```python
from build123d import *

# Parameters (mm, degrees)
SKETCH1_W           = 150
SKETCH1_H           = 40
BOSS_EXTRUDE1_DEPTH = 2
SKETCH2_W           = 150
SKETCH2_H           = 2
BOSS_EXTRUDE2_DEPTH = 40
BOSS_EXTRUDE3_DEPTH = 390
CUT_EXTRUDE1_DEPTH  = 10
CUT_EXTRUDE2_DEPTH  = 10


with BuildPart() as part:
    # Sketch1 → Boss-Extrude1 (new body)
    with BuildSketch(Plane(origin=(0, 0, 0), x_dir=(1, 0, 0), z_dir=(0, 1, 0))):
        Rectangle(SKETCH1_W, SKETCH1_H)
    extrude(amount=BOSS_EXTRUDE1_DEPTH)

    # Sketch2 → Boss-Extrude2 (add)
    with BuildSketch(Plane(origin=(0, 2, 0), x_dir=(1, 0, 0), z_dir=(0, 1, 0))):
        with Locations((0, -19)):
            Rectangle(SKETCH2_W, SKETCH2_H)
    extrude(amount=BOSS_EXTRUDE2_DEPTH)

    # Sketch5 → Boss-Extrude3 (add)
    with BuildSketch(Plane(origin=(75, 0, 0), x_dir=(0, 0, -1), z_dir=(1, 0, 0))):
        Polygon((-20, 0), (20, 0), (20, 2), (-18, 2), (-18, 42), (-20, 42), align=None)
    extrude(amount=BOSS_EXTRUDE3_DEPTH)

    # Sketch6 → Cut-Extrude1 (cut)
    with BuildSketch(Plane.XZ):
        with BuildLine():
            Line((7.420621343, 6.493750786), (43.697093864, 6.493750786))
            ThreePointArc((43.697093864, 6.493750786), (50.190844651, 0), (43.697093864, -6.493750786))
            Line((43.697093864, -6.493750786), (7.420621343, -6.493750786))
            ThreePointArc((7.420621343, -6.493750786), (0.926870557, 0), (7.420621343, 6.493750786))
        make_face()
        with BuildLine():
            Line((-57.579378657, 6.493750786), (-21.302906136, 6.493750786))
            ThreePointArc((-21.302906136, 6.493750786), (-14.809155349, 0), (-21.302906136, -6.493750786))
            Line((-21.302906136, -6.493750786), (-57.579378657, -6.493750786))
            ThreePointArc((-57.579378657, -6.493750786), (-64.073129443, 0), (-57.579378657, 6.493750786))
        make_face()
        with BuildLine():
            Line((72.420621343, 6.493750786), (108.697093864, 6.493750786))
            ThreePointArc((108.697093864, 6.493750786), (115.190844651, 0), (108.697093864, -6.493750786))
            Line((108.697093864, -6.493750786), (72.420621343, -6.493750786))
            ThreePointArc((72.420621343, -6.493750786), (65.926870557, 0), (72.420621343, 6.493750786))
        make_face()
        with BuildLine():
            Line((137.420621343, 6.493750786), (173.697093864, 6.493750786))
            ThreePointArc((173.697093864, 6.493750786), (180.190844651, 0), (173.697093864, -6.493750786))
            Line((173.697093864, -6.493750786), (137.420621343, -6.493750786))
            ThreePointArc((137.420621343, -6.493750786), (130.926870557, 0), (137.420621343, 6.493750786))
        make_face()
        with BuildLine():
            Line((202.420621343, 6.493750786), (238.697093864, 6.493750786))
            ThreePointArc((238.697093864, 6.493750786), (245.190844651, 0), (238.697093864, -6.493750786))
            Line((238.697093864, -6.493750786), (202.420621343, -6.493750786))
            ThreePointArc((202.420621343, -6.493750786), (195.926870557, 0), (202.420621343, 6.493750786))
        make_face()
        with BuildLine():
            Line((267.420621343, 6.493750786), (303.697093864, 6.493750786))
            ThreePointArc((303.697093864, 6.493750786), (310.190844651, 0), (303.697093864, -6.493750786))
            Line((303.697093864, -6.493750786), (267.420621343, -6.493750786))
            ThreePointArc((267.420621343, -6.493750786), (260.926870557, 0), (267.420621343, 6.493750786))
        make_face()
        with BuildLine():
            Line((332.420621343, 6.493750786), (368.697093864, 6.493750786))
            ThreePointArc((368.697093864, 6.493750786), (375.190844651, 0), (368.697093864, -6.493750786))
            Line((368.697093864, -6.493750786), (332.420621343, -6.493750786))
            ThreePointArc((332.420621343, -6.493750786), (325.926870557, 0), (332.420621343, 6.493750786))
        make_face()
        with BuildLine():
            Line((397.420621343, 6.493750786), (433.697093864, 6.493750786))
            ThreePointArc((433.697093864, 6.493750786), (440.190844651, 0), (433.697093864, -6.493750786))
            Line((433.697093864, -6.493750786), (397.420621343, -6.493750786))
            ThreePointArc((397.420621343, -6.493750786), (390.926870557, 0), (397.420621343, 6.493750786))
        make_face()
    extrude(amount=-CUT_EXTRUDE1_DEPTH, mode=Mode.SUBTRACT)

    # Sketch7 → Cut-Extrude2 (cut)
    with BuildSketch(Plane.XY.offset(20)):
        with BuildLine():
            Line((-2.201358411, 29.022590271), (32.798641589, 29.022590271))
            ThreePointArc((32.798641589, 29.022590271), (40.548675365, 21.272556495), (32.798641589, 13.522522718))
            Line((32.798641589, 13.522522718), (-2.201358411, 13.522522718))
            ThreePointArc((-2.201358411, 13.522522718), (-9.951392188, 21.272556495), (-2.201358411, 29.022590271))
        make_face()
        with BuildLine():
            Line((-59.201358411, 29.022590271), (-24.201358411, 29.022590271))
            ThreePointArc((-24.201358411, 29.022590271), (-16.451324635, 21.272556495), (-24.201358411, 13.522522718))
            Line((-24.201358411, 13.522522718), (-59.201358411, 13.522522718))
            ThreePointArc((-59.201358411, 13.522522718), (-66.951392188, 21.272556495), (-59.201358411, 29.022590271))
        make_face()
        with BuildLine():
            Line((54.798641589, 29.022590271), (89.798641589, 29.022590271))
            ThreePointArc((89.798641589, 29.022590271), (97.548675365, 21.272556495), (89.798641589, 13.522522718))
            Line((89.798641589, 13.522522718), (54.798641589, 13.522522718))
            ThreePointArc((54.798641589, 13.522522718), (47.048607812, 21.272556495), (54.798641589, 29.022590271))
        make_face()
        with BuildLine():
            Line((111.798641589, 29.022590271), (146.798641589, 29.022590271))
            ThreePointArc((146.798641589, 29.022590271), (154.548675365, 21.272556495), (146.798641589, 13.522522718))
            Line((146.798641589, 13.522522718), (111.798641589, 13.522522718))
            ThreePointArc((111.798641589, 13.522522718), (104.048607812, 21.272556495), (111.798641589, 29.022590271))
        make_face()
        with BuildLine():
            Line((168.798641589, 29.022590271), (203.798641589, 29.022590271))
            ThreePointArc((203.798641589, 29.022590271), (211.548675365, 21.272556495), (203.798641589, 13.522522718))
            Line((203.798641589, 13.522522718), (168.798641589, 13.522522718))
            ThreePointArc((168.798641589, 13.522522718), (161.048607812, 21.272556495), (168.798641589, 29.022590271))
        make_face()
        with BuildLine():
            Line((225.798641589, 29.022590271), (260.798641589, 29.022590271))
            ThreePointArc((260.798641589, 29.022590271), (268.548675365, 21.272556495), (260.798641589, 13.522522718))
            Line((260.798641589, 13.522522718), (225.798641589, 13.522522718))
            ThreePointArc((225.798641589, 13.522522718), (218.048607812, 21.272556495), (225.798641589, 29.022590271))
        make_face()
        with BuildLine():
            Line((282.798641589, 29.022590271), (317.798641589, 29.022590271))
            ThreePointArc((317.798641589, 29.022590271), (325.548675365, 21.272556495), (317.798641589, 13.522522718))
            Line((317.798641589, 13.522522718), (282.798641589, 13.522522718))
            ThreePointArc((282.798641589, 13.522522718), (275.048607812, 21.272556495), (282.798641589, 29.022590271))
        make_face()
        with BuildLine():
            Line((339.798641589, 29.022590271), (374.798641589, 29.022590271))
            ThreePointArc((374.798641589, 29.022590271), (382.548675365, 21.272556495), (374.798641589, 13.522522718))
            Line((374.798641589, 13.522522718), (339.798641589, 13.522522718))
            ThreePointArc((339.798641589, 13.522522718), (332.048607812, 21.272556495), (339.798641589, 29.022590271))
        make_face()
        with BuildLine():
            Line((396.798641589, 29.022590271), (431.798641589, 29.022590271))
            ThreePointArc((431.798641589, 29.022590271), (439.548675365, 21.272556495), (431.798641589, 13.522522718))
            Line((431.798641589, 13.522522718), (396.798641589, 13.522522718))
            ThreePointArc((396.798641589, 13.522522718), (389.048607812, 21.272556495), (396.798641589, 29.022590271))
        make_face()
    extrude(amount=-CUT_EXTRUDE2_DEPTH, mode=Mode.SUBTRACT)


solid = part.part
```
Could you check a few things on this model? Use its own coordinates, in mm. A direction names the side the tool comes from. Coordinates: 2 decimals unless noted, no trailing zeros. Loops run counter-clockwise (first coordinate to the right, second up) from the corner with the lowest first, then second, coordinate; pieces in that order, holes last. Notation, with made-up numbers: M 81,-25 L 111,-25 A24 ccw 111,9 Z; hole C 28,-15 d1. An arc over 180 degrees is marked long. Put each result on its own line as item: value. Start each with the question number.
(1) For faces 1 (the face through (191, 13, 18)), 2 (the face through (191, 0, 0)), which set-ups out of +Z, -Z, +X, -X, +Y, -Y let a thin tool reach every point of the face, with its end or its side?
(2) Will these pins go through, and if not, where does the flat tip stop? P1, Ø19, axis at x = 302.5, z = 0.5, coming from the +Y side; P2, Ø2, axis at x = 361.5, z = 19.5, coming from the -Y side; P3, Ø20, axis at x = 223.5, y = 16.5, coming from the -Z side.
(3) Suppose I cut it at B-B on y = 7.5. Please give me the cut outline in (x, z), then the cut area to 3 significant figures.
(4) Suppose I cut it at C-C on z = 0. Count the separate pieces of the cut face and the enclosed holes in it, then the cut area to 3 significant figures.
(5) Suppose I cut it at A-A on x = -40.5. Please give me the cut outline in (y, z).
(6) I need wall thicknesses on line 1 (Y direction, x = 67, z = -10); line 2 (Z direction, x = 107, y = 10). Which ranges of each line are inside material? Lowest first, please. Write a range as from..to.
Solutions:
1. face 1: -Z, +X, -X, +Y
1. face 2: +Z, -Z, +X, -X, -Y
2. P1: stops at y = 2
2. P2: stops at y = 0
2. P3: stops at z = 18
3. outline: M -75,18 L 465,18 L 465,20 L -75,20 Z
3. area: 1,080 mm2
4. separate pieces: 9
4. enclosed holes: 0
4. area: 292 mm2
5. outline: M 0,-20 L 2,-20 L 2,-6.49 L 0,-6.49 Z; M 0,6.49 L 2,6.49 L 2,18 L 13.52,18 L 13.52,20 L 0,20 Z; M 29.02,18 L 42,18 L 42,20 L 29.02,20 Z
6. line 1: y = 0..2
6. line 2: z = 18..20
